```python
from build123d import *

# Parameters (mm, degrees)
F0_W     = 88.9
F0_H     = 88.9
F1_DEPTH = 673.1
F2_W     = 88.9
F2_H     = 44.45
F3_DEPTH = 88.901
F5_DEPTH = 1346.201
F6_W     = 88.9
F6_H     = 88.9
F7_DEPTH = 88.901


with BuildPart() as f1:
    # F0 (on Right) → F1 (new body, symmetric)
    with BuildSketch(Plane.YZ):
        Rectangle(F0_W, F0_H)
    extrude(amount=F1_DEPTH, both=True)

    # F2 (on face) → F3 (cut, through all)
    with BuildSketch(Plane.XZ.offset(44.45)):
        with Locations((-539.75, 22.225)):
            Rectangle(F2_W, F2_H)
        with Locations((539.75, 22.225)):
            Rectangle(F2_W, F2_H)
    extrude(amount=-F3_DEPTH, mode=Mode.SUBTRACT)

    # F4 (on face) → F5 (cut, through all)
    with BuildSketch(Plane.YZ.offset(673.1)):
        Polygon((44.45, -44.45), (44.45, 44.45), (28.774531, -44.45), align=None)
    extrude(amount=-F5_DEPTH, mode=Mode.SUBTRACT)

    # F6 (on face) → F7 (cut, through all)
    with BuildSketch(Plane.XZ.offset(44.45)):
        with Locations((-628.65, 0)):
            Rectangle(F6_W, F6_H)
        with Locations((628.65, 0)):
            Rectangle(F6_W, F6_H)
    extrude(amount=-F7_DEPTH, mode=Mode.SUBTRACT)


solid = f1.part
```
Check sheet for the modelled part. Datum: model origin and axes. Units: mm. A direction names the side the tool comes from. Round coordinates to 2 decimals unless told otherwise and drop trailing zeros. Loops run counter-clockwise (first coordinate to the right, second up) from the corner with the lowest first, then second, coordinate; pieces in that order, holes last. Notation, with made-up numbers: (17.25, 84.5) - (59.25, 84.5) arc R7 cw to (59.25, 93.5) - close; hole circle Ø4 at (37.25, 26). An arc over 180 degrees is marked (long way). Answer as a JSON object with one key per item and string values. Group by question number.
Q1. Set-up check for faces 1 (the face through (-540, -4, 0)), 2 (the face through (7, -1, 44.45)), 3 (the face through (539, -4, 0)): record each of +Z, -Z, +X, -X, +Y, -Y from which the full face is reachable in a straight line by a thin tool's end or side.
Q2. Sectioned sample at A-A, the plane y = -27. Enter the section's corners in (x, z).
Q3. Sectioned sample at B-B, the plane x = -153.5. Enter the section's corners in (y, z).
Q4. Scan lines: line 1 along Y through (x, z) = (-313, -0.5); line 2 along X through (y, z) = (-1.5, 13); line 3 along Y through (x, z) = (-269.5, -1.5). Record each from-to range of solid material in increasing order. Write a range as [from, to].
Q5. Mould release check, pull along Y, two halves, no side actions. Record for faces 4 (the face through (8.18, 36.72, 0.62)), 5 (the face through (-584.2, -4, -23)), 6 (the face through (8, -44.45, -1)): released by +Y, released by -Y, zero draft, split by the parting line, or undercut.
Q6. Gauge pin test, flat ends, axial feed: P1, Ø8, axis at x = -173, z = -22.5, coming from the +Y side; P2, Ø12, axis at x = -263, z = -13, coming from the +Y side. Record the tip position at first contact, or that the pin passes through.
Q7. Sectioned sample at C-C, the plane z = 12. Enter the section's corners in (x, y).
Solution:
{
 "1": {"face 1": "+Z, -X, +Y, -Y", "face 2": "+Z, +X, -X, +Y, -Y", "face 3": "+Z, +X, +Y, -Y"},
 "2": {"outline": "(-584.2, -44.45) - (584.2, -44.45) - (584.2, 0) - (495.3, 0) - (495.3, 44.45) - (-495.3, 44.45) - (-495.3, 0) - (-584.2, 0) - close"},
 "3": {"outline": "(-44.45, -44.45) - (28.77, -44.45) - (44.45, 44.45) - (-44.45, 44.45) - close"},
 "4": {"line 1": "y = [-44.45, 36.52]", "line 2": "x = [-495.3, 495.3]", "line 3": "y = [-44.45, 36.35]"},
 "5": {"face 4": "released by +Y", "face 5": "zero draft", "face 6": "released by -Y"},
 "6": {"P1": "stops at y = 33.35", "P2": "stops at y = 35.38"},
 "7": {"outline": "(-495.3, -44.45) - (495.3, -44.45) - (495.3, 38.73) - (-495.3, 38.73) - close"}
}
